```python
from build123d import *

# Parameters (mm, degrees)
SKETCH1_W           = 120
SKETCH1_H           = 100
BOSS_EXTRUDE1_DEPTH = 50
SKETCH2_W           = 112
SKETCH2_H           = 92
CUT_EXTRUDE1_DEPTH  = 46
SKETCH3_W           = 24.6
SKETCH3_H           = 70
BOSS_EXTRUDE3_DEPTH = 8
SKETCH6_W           = 24.61
SKETCH6_H           = 8
CUT_EXTRUDE4_DEPTH  = 66
SKETCH7_W           = 26
SKETCH7_H           = 10
CUT_EXTRUDE6_DEPTH  = 66
SKETCH10_R          = 9
CUT_EXTRUDE9_DEPTH  = 12.5
SKETCH8_R           = 11.662197426
CUT_EXTRUDE10_DEPTH = 10


with BuildPart() as part:
    # Sketch1 → Boss-Extrude1 (new body)
    with BuildSketch(Plane(origin=(0, 0, 0), x_dir=(1, 0, 0), z_dir=(0, 1, 0))):
        with Locations((-10.571222942, 10.082692781)):
            Rectangle(SKETCH1_W, SKETCH1_H)
    extrude(amount=BOSS_EXTRUDE1_DEPTH)

    # Sketch2 → Cut-Extrude1 (cut)
    with BuildSketch(Plane(origin=(0, 50, 0), x_dir=(1, 0, 0), z_dir=(0, 1, 0))):
        with Locations((-10.571222942, 10.082692781)):
            Rectangle(SKETCH2_W, SKETCH2_H)
    extrude(amount=-CUT_EXTRUDE1_DEPTH, mode=Mode.SUBTRACT)

    # Sketch3 → Boss-Extrude3 (add)
    with BuildSketch(Plane(origin=(0, 4, 0), x_dir=(1, 0, 0), z_dir=(0, 1, 0))):
        with Locations((-44.271222942, 25.082692781)):
            Rectangle(SKETCH3_W, SKETCH3_H)
    extrude(amount=BOSS_EXTRUDE3_DEPTH)

    # Sketch6 → Cut-Extrude4 (cut)
    with BuildSketch(Plane.XY.offset(9.917307219)):
        with Locations((-42.369304131, 8)):
            Rectangle(SKETCH6_W, SKETCH6_H)
    extrude(amount=-CUT_EXTRUDE4_DEPTH, mode=Mode.SUBTRACT)

    # Sketch7 → Cut-Extrude6 (cut)
    with BuildSketch(Plane.XY.offset(-56.082692781)):
        with Locations((-41.674304131, 9)):
            Rectangle(SKETCH7_W, SKETCH7_H)
    extrude(amount=-CUT_EXTRUDE6_DEPTH, mode=Mode.SUBTRACT)

    # Sketch10 → Cut-Extrude9 (cut)
    with BuildSketch(Plane(origin=(0, 0, -60.082692781), x_dir=(-1, 0, 0), z_dir=(0, 0, -1))):
        with Locations((-27.728777058, 25)):
            Circle(SKETCH10_R)
    extrude(amount=-CUT_EXTRUDE9_DEPTH, mode=Mode.SUBTRACT)

    # Sketch8 → Cut-Extrude10 (cut)
    with BuildSketch(Plane.XY.offset(-56.082692781)):
        with Locations((0.428777058, 24)):
            Circle(SKETCH8_R)
    extrude(amount=-CUT_EXTRUDE10_DEPTH, mode=Mode.SUBTRACT)


solid = part.part
```
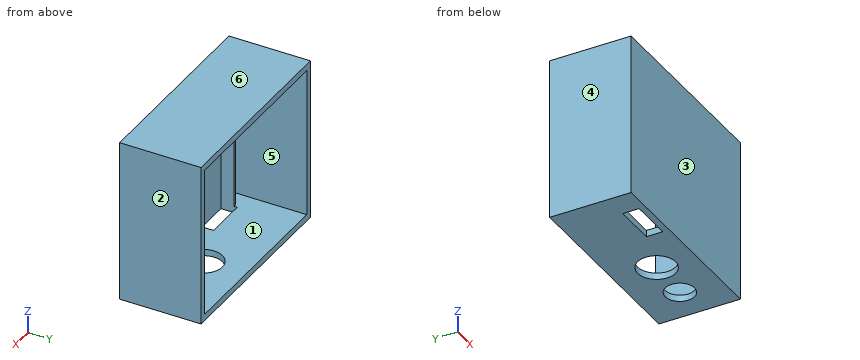
CAD build for the part. Positions are in the model's coordinates, mm. Face numbers are marked on the shaded views. A direction names the side the tool comes from. Round coordinates to 2 decimals unless told otherwise and drop trailing zeros. Write each loop counter-clockwise with the first axis right and the second up, starting at its lowest first coordinate (ties: lowest second). Pieces come first, ordered by that corner, then holes. Notation, with made-up numbers: (-25, -9.75) -> (7, -9.75) arc R24 cw to (7, 17.25) -> close; hole circle Ø2 at (39, 36.5). An arc over 180 degrees is marked (long way). Answer in a Markdown table with one row per item. Add a question column.
Item 1: Drop flat-ended pins along their axis: pin 1 Ø1.5 at (x, z) = (-55.5, -28.5) entering from +Y; pin 2 Ø2 at (x, z) = (-24.5, -15.5) entering from +Y. Give the stop position or say it passes through.
Item 2: Mould opens along X. For the marked faces 1, 2, 3 and 4 say: pulls with the +X half, pulls with the -X half, needs draft (parallel to the pull), parting line crosses it, or undercut.
Item 3: Saw through at D-D, the plane z = 1. Write the cut outline in (x, y).
Item 4: Saw through at C-C, the plane x = -15. Write the cut outline in (y, z), then the cut area to 3 significant figures.
Item 5: Saw through at B-B, the plane y = 44. Write the cut outline in (x, z).
Item 6: Which spindle directions (+Z, -Z, +X, -X, +Y, -Y) get a long thin tool onto all of the face, cutting with end or side? Do the marked faces 5 and 6. Say none if no direction does.
Item 7: Saw through at A-A, the plane x = -49.5. Write the cut outline in (y, z).
Item 8: Drill centre lines: line 1 (X direction, y = 8, z = -27.5); line 2 (Z direction, x = -64, y = 39); line 3 (X direction, y = 22, z = -21.5). Where is each one in solid material? Low to high. Write a range as from..to.
Findings below:
| question | item | result |
|---|---|---|
| 1 | pin 1 | stops at y = 12 |
| 1 | pin 2 | stops at y = 4 |
| 2 | face 1 | undercut |
| 2 | face 2 | pulls with the +X half |
| 2 | face 3 | needs draft |
| 2 | face 4 | pulls with the -X half |
| 3 | outline | (-70.57, 0) -> (49.43, 0) -> (49.43, 50) -> (45.43, 50) -> (45.43, 4) -> (-54.67, 4) -> (-54.67, 12) -> (-56.57, 12) -> (-56.57, 4) -> (-66.57, 4) -> (-66.57, 50) -> (-70.57, 50) -> close |
| 4 | outline | (0, -60.08) -> (50, -60.08) -> (50, -56.08) -> (4, -56.08) -> (4, 35.92) -> (50, 35.92) -> (50, 39.92) -> (0, 39.92) -> close |
| 4 | area | 768 mm^2 |
| 5 | outline | (-70.57, -60.08) -> (49.43, -60.08) -> (49.43, 39.92) -> (-70.57, 39.92) -> close; hole (-66.57, -56.08) -> (45.43, -56.08) -> (45.43, 35.92) -> (-66.57, 35.92) -> close |
| 6 | face 5 | +Y |
| 6 | face 6 | +Z, +X, -X, +Y, -Y |
| 7 | outline | (0, -60.08) -> (4, -60.08) -> (4, 35.92) -> (50, 35.92) -> (50, 39.92) -> (0, 39.92) -> close; (14, -60.08) -> (50, -60.08) -> (50, -56.08) -> (14, -56.08) -> close |
| 8 | line 1 | x = -70.57..-66.57, -56.57..-54.67, 45.43..49.43 |
| 8 | line 2 | z = -60.08..-56.08, 35.92..39.92 |
| 8 | line 3 | x = -70.57..-66.57, 45.43..49.43 |
